Could you check a few things on this model? Use its own coordinates, in mm. Face numbers are marked on the shaded views. A direction names the side the tool comes from. Give positions to 0.01 mm unless a question says otherwise; leave off trailing zeros. Order: outer loops, then holes, each group sorted by start corner. A loop starts at its lowest first (then second) coordinate and runs counter-clockwise, first axis right, second up.
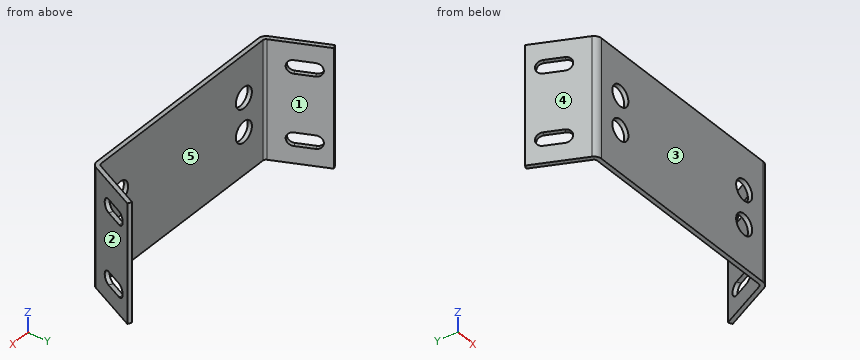
from build123d import *

# Parameters (mm, degrees)
BASE_FLANGE1_DEPTH = 31.75
CUT_EXTRUDE1_REACH = 86.256
SKETCH3_R          = 5.5626
CUT_EXTRUDE2_REACH = 137.032


# Sheet-metal steps are written as plain solids
with BuildPart() as part:
    # Sketch1 → Base-Flange1 (new, symmetric)
    with BuildSketch(Plane.XY):
        with BuildLine():
            Line((-72.15562981, 28.775272238), (-59.81800404, 2.317148392))
            ThreePointArc((-59.81800404, 2.317148392), (-58.337100418, 0.62850145), (-56.180809629, 0))
            Line((-56.180809629, 0), (56.180809629, 0))
            ThreePointArc((56.180809629, 0), (58.337100418, 0.62850145), (59.81800404, 2.317148392))
            Line((59.81800404, 2.317148392), (72.15562981, 28.775272238))
            Line((72.15562981, 28.775272238), (70.083810209, 29.741377585))
            Line((70.083810209, 29.741377585), (57.746184439, 3.283253738))
            ThreePointArc((57.746184439, 3.283253738), (57.108833513, 2.556494295), (56.180809629, 2.286))
            Line((56.180809629, 2.286), (-56.180809629, 2.286))
            ThreePointArc((-56.180809629, 2.286), (-57.108833513, 2.556494295), (-57.746184439, 3.283253738))
            Line((-57.746184439, 3.283253738), (-70.083810209, 29.741377585))
            Line((-70.083810209, 29.741377585), (-72.15562981, 28.775272238))
        make_face()
    extrude(amount=BASE_FLANGE1_DEPTH, both=True)

    # Sketch3 → Cut-Extrude1 (cut, up to next)
    with BuildSketch(Plane(origin=(0, 0, 0), x_dir=(1, 0, 0), z_dir=(0, 1, 0)), mode=Mode.PRIVATE) as cut_extrude1_sk1:
        with Locations(Location((43, 9, 0), (0, 0, 90))):
            Circle(SKETCH3_R)
    cut_extrude1_tool1 = extrude(cut_extrude1_sk1.sketch, amount=CUT_EXTRUDE1_REACH, mode=Mode.PRIVATE) & part.part
    # Sketch3 → Cut-Extrude1 (cut, up to next)
    with BuildSketch(Plane(origin=(0, 0, 0), x_dir=(1, 0, 0), z_dir=(0, 1, 0)), mode=Mode.PRIVATE) as cut_extrude1_sk2:
        with Locations(Location((43, -9, 0), (0, 0, 90))):
            Circle(SKETCH3_R)
    cut_extrude1_tool2 = extrude(cut_extrude1_sk2.sketch, amount=CUT_EXTRUDE1_REACH, mode=Mode.PRIVATE) & part.part
    # Sketch3 → Cut-Extrude1 (cut, up to next)
    with BuildSketch(Plane(origin=(0, 0, 0), x_dir=(1, 0, 0), z_dir=(0, 1, 0)), mode=Mode.PRIVATE) as cut_extrude1_sk3:
        with Locations(Location((-43, -9, 0), (0, 0, 90))):
            Circle(SKETCH3_R)
    cut_extrude1_tool3 = extrude(cut_extrude1_sk3.sketch, amount=CUT_EXTRUDE1_REACH, mode=Mode.PRIVATE) & part.part
    # Sketch3 → Cut-Extrude1 (cut, up to next)
    with BuildSketch(Plane(origin=(0, 0, 0), x_dir=(1, 0, 0), z_dir=(0, 1, 0)), mode=Mode.PRIVATE) as cut_extrude1_sk4:
        with Locations(Location((-43, 9, 0), (0, 0, 90))):
            Circle(SKETCH3_R)
    cut_extrude1_tool4 = extrude(cut_extrude1_sk4.sketch, amount=CUT_EXTRUDE1_REACH, mode=Mode.PRIVATE) & part.part
    add(cut_extrude1_tool1.solids().sort_by_distance((43, 0, -9))[0], mode=Mode.SUBTRACT)
    add(cut_extrude1_tool2.solids().sort_by_distance((43, 0, 9))[0], mode=Mode.SUBTRACT)
    add(cut_extrude1_tool3.solids().sort_by_distance((-43, 0, 9))[0], mode=Mode.SUBTRACT)
    add(cut_extrude1_tool4.solids().sort_by_distance((-43, 0, -9))[0], mode=Mode.SUBTRACT)

    # Sketch4 → Cut-Extrude2 (cut, up to next)
    with BuildSketch(Plane(origin=(48.246618612, -22.497767739, 0), x_dir=(0, 0, -1), z_dir=(0.9063077870366514, -0.4226182617406968, 0)), mode=Mode.PRIVATE) as cut_extrude2_sk1:
        with BuildLine():
            Line((22.6187, 39.098340149), (22.6187, 48.623340149))
            ThreePointArc((22.6187, 48.623340149), (19.05, 52.192040149), (15.4813, 48.623340149))
            Line((15.4813, 48.623340149), (15.4813, 39.098340149))
            ThreePointArc((15.4813, 39.098340149), (19.05, 35.529640149), (22.6187, 39.098340149))
        make_face()
    cut_extrude2_tool1 = extrude(cut_extrude2_sk1.sketch, amount=-CUT_EXTRUDE2_REACH, mode=Mode.PRIVATE) & part.part
    # Sketch4 → Cut-Extrude2 (cut, up to next)
    with BuildSketch(Plane(origin=(48.246618612, -22.497767739, 0), x_dir=(0, 0, -1), z_dir=(0.9063077870366514, -0.4226182617406968, 0)), mode=Mode.PRIVATE) as cut_extrude2_sk2:
        with BuildLine():
            Line((-15.4813, 48.623340149), (-15.4813, 39.098340149))
            ThreePointArc((-15.4813, 39.098340149), (-19.05, 35.529640149), (-22.6187, 39.098340149))
            Line((-22.6187, 39.098340149), (-22.6187, 48.623340149))
            ThreePointArc((-22.6187, 48.623340149), (-19.05, 52.192040149), (-15.4813, 48.623340149))
        make_face()
    cut_extrude2_tool2 = extrude(cut_extrude2_sk2.sketch, amount=-CUT_EXTRUDE2_REACH, mode=Mode.PRIVATE) & part.part
    cut_extrude2_1 = cut_extrude2_tool1.solids().sort_by_distance((66.783011, 17.253653, -19.05))[0]
    add(cut_extrude2_1, mode=Mode.SUBTRACT)
    cut_extrude2_2 = cut_extrude2_tool2.solids().sort_by_distance((66.783011, 17.253653, 19.05))[0]
    add(cut_extrude2_2, mode=Mode.SUBTRACT)
    cut_extrude2 = cut_extrude2_1 + cut_extrude2_2  # Cut-Extrude2 as one shape, for the pattern or mirror that repeats it

    # Mirror1: Cut-Extrude2 across plane
    add(cut_extrude2.mirror(Plane(origin=(0, 0, 0), x_dir=(0, 0, 1), z_dir=(1, 0, 0))), mode=Mode.SUBTRACT)


solid = part.part
Item 1: Imagine slicing it at C-C on y = 15.5. List the corners of the cut face in (x, z) for me, then the cut area to 3 significant figures.
Findings:
outline: (-65.97, -31.75) - (-63.44, -31.75) - (-63.44, -22.62) - (-65.97, -22.62) - close; (-65.97, -15.48) - (-63.44, -15.48) - (-63.44, 15.48) - (-65.97, 15.48) - close; (-65.97, 22.62) - (-63.44, 22.62) - (-63.44, 31.75) - (-65.97, 31.75) - close; (63.44, -31.75) - (65.97, -31.75) - (65.97, -22.62) - (63.44, -22.62) - close; (63.44, -15.48) - (65.97, -15.48) - (65.97, 15.48) - (63.44, 15.48) - close; (63.44, 22.62) - (65.97, 22.62) - (65.97, 31.75) - (63.44, 31.75) - close
area: 248 mm2
Item 2: Imagine slicing it at B-B on x = -43. List the corners of the cut face in (y, z) for me, then the cut area to 3 significant figures.
Findings:
outline: (0, -31.75) - (2.29, -31.75) - (2.29, -14.56) - (0, -14.56) - close; (0, -3.44) - (2.29, -3.44) - (2.29, 3.44) - (0, 3.44) - close; (0, 14.56) - (2.29, 14.56) - (2.29, 31.75) - (0, 31.75) - close
area: 94.3 mm2
Item 3: For pin 1 (8 mm diameter, centred on x = 9, z = 18.5, fed in from +Y); pin 2 (8 mm diameter, centred on y = 5.5, z = -7.5, fed in from -X), each with a flat end and sliding along its axis, tell me the tip position at first contact or that it passes through.
Findings:
pin 1: stops at y = 2.29
pin 2: stops at x = -63.17
Item 4: Please list where these lines run through material, in increasing order: line 1 along Z through (x, y) = (-43, 1.6); line 2 along X through (y, z) = (1.35, 9); line 3 along X through (y, z) = (1.7, 9).
Findings:
line 1: z = -31.75 to -14.56, -3.44 to 3.44, 14.56 to 31.75
line 2: x = -59.18 to -48.56, -37.44 to 37.44, 48.56 to 59.18
line 3: x = -59.46 to -48.56, -37.44 to 37.44, 48.56 to 59.46
Item 5: We'd pull the mould along X, two halves only. Please class the marked faces 3, 4 and 5: +X half, -X half, draft (parallel to the pull), parting line (faces both ways), or undercut.
Findings:
face 3: draft
face 4: -X half
face 5: undercut
Item 6: Imagine slicing it at D-D on z = 25. List the corners of the cut face in (x, y) for me.
Findings:
outline: (-72.16, 28.78) - (-59.82, 2.32) arc R4.01 ccw to (-56.18, 0) - (56.18, 0) arc R4.01 ccw to (59.82, 2.32) - (72.16, 28.78) - (70.08, 29.74) - (57.75, 3.28) arc R1.73 cw to (56.18, 2.29) - (-56.18, 2.29) arc R1.73 cw to (-57.75, 3.28) - (-70.08, 29.74) - close
Item 7: Imagine slicing it at A-A on z = -9. List the corners of the cut face in (x, y) for me, then the cut area to 3 significant figures.
Findings:
outline: (-72.16, 28.78) - (-59.82, 2.32) arc R4.01 ccw to (-56.18, 0) - (-48.56, 0) - (-48.56, 2.29) - (-56.18, 2.29) arc R1.73 cw to (-57.75, 3.28) - (-70.08, 29.74) - close; (-37.44, 0) - (37.44, 0) - (37.44, 2.29) - (-37.44, 2.29) - close; (48.56, 0) - (56.18, 0) arc R4.01 ccw to (59.82, 2.32) - (72.16, 28.78) - (70.08, 29.74) - (57.75, 3.28) arc R1.73 cw to (56.18, 2.29) - (48.56, 2.29) - close
area: 354 mm2
Item 8: For the marked faces 1 and 2, which set-ups out of +Z, -Z, +X, -X, +Y, -Y let a thin tool reach every point of the face, with its end or its side?
Findings:
face 1: +Z, -Z, +Y
face 2: +Z, -Z, +X, -Y
